Geometry: final body of the model. Coordinates: model frame, mm. A direction names the side the tool comes from. Round coordinates to 2 decimals unless told otherwise and drop trailing zeros. Loops run counter-clockwise (first coordinate to the right, second up) from the corner with the lowest first, then second, coordinate; pieces in that order, holes last. Notation, with made-up numbers: (74, 0) -> (102, 0) arc R16 ccw to (102, 12) -> close; hole circle Ø6 at (4, 66). An arc over 180 degrees is marked (long way). Answer in a Markdown table with one row per item.
Autodesk Inventor part; units mm, degrees
ref_plane "YZ Plane" through (0, 0, 0) normal (1, 0, 0) x (0, 1, 0)
ref_plane "XZ Plane" through (0, 0, 0) normal (0, 1, 0) x (-1, 0, 0)
ref_plane "XY Plane" through (0, 0, 0) normal (0, 0, 1) x (1, 0, 0)
sketch "Sketch_15" plane through (0, 0, 0) normal (1, 0, 0) x (0, 1, 0)
  line L0 (0, 30) -> (0, 0)
  line L1 (0, 0) -> (30, 0)
  line L2 (30, 0) -> (30, 4.0858)
  arc A0 (30, 4.0858) -> (29.7071, 4.7929) centre (29, 4.0858) ccw
  line L3 (29.7071, 4.7929) -> (4.7929, 29.7071)
  arc A1 (4.7929, 29.7071) -> (4.0858, 30) centre (4.0858, 29) ccw
  line L4 (4.0858, 30) -> (0, 30)
extrude "Extrusion1" add sketch "Sketch_15" along normal mid plane 20
sketch "Sketch_16" plane through (0, 0, 0) normal (1, 0, 0) x (0, 1, 0)
  line L0 (2.9278, 34.5) -> (4.5, 4.5)
  line L1 (4.5, 4.5) -> (34.5, 4.5)
  line L2 (34.5, 4.5) -> (34.5, 34.5)
  line L3 (34.5, 34.5) -> (2.9278, 34.5)
extrude "Extrusion2" cut sketch "Sketch_16" along normal mid plane 15
sketch "Sketch_17" plane through (0, 4.5, 0) normal (0, 1, 0) x (1, 0, 0)
  line L0 (-5.4209, -10.5) -> (-4.4687, -18.5299)
  arc A0 (-4.4687, -18.5299) -> (4.4687, -18.5299) centre (0, -18) ccw
  line L1 (4.4687, -18.5299) -> (5.4209, -10.5)
  line L2 (5.4209, -10.5) -> (-5.4209, -10.5)
extrude "Extrusion3" add sketch "Sketch_17" against normal blind 2.25
sketch "Sketch_2" plane through (0, 0, 0) normal (0, 0, 1) x (1, 0, 0)
  circle A0 centre (0, 18) radius 2.1
extrude "Extrusion4" cut sketch "Sketch_2" along normal blind 4.5
sketch "Sketch_9" plane through (0, 0, 0) normal (0, 0, 1) x (1, 0, 0)
  circle A0 centre (0, 10) radius 2.1
extrude "Extrusion5" cut sketch "Sketch_9" along normal blind 4.5
sketch "Sketch_3" plane through (0, 0, 0) normal (0, 1, 0) x (-1, 0, 0)
  circle A0 centre (0, 18) radius 2.1
extrude "Extrusion6" cut sketch "Sketch_3" along normal blind 4.5
sketch "Sketch_1" plane through (0, 0, 0) normal (0, 1, 0) x (-1, 0, 0)
  line L0 (10, 0) -> (10, 30)
  line L1 (10, 30) -> (-10, 30)
  line L2 (-10, 30) -> (-10, 0)
  line L3 (-10, 0) -> (10, 0)
extrude "Extrusion7" add sketch "Sketch_1" against normal blind 1
sketch "Sketch_4" plane through (0, 0, 0) normal (0, 1, 0) x (-1, 0, 0)
  line L0 (10, 0) -> (10, 30)
  line L1 (10, 30) -> (-10, 30)
  line L2 (-10, 30) -> (-10, 0)
  line L3 (-10, 0) -> (10, 0)
  arc A0 (3, 10.7) -> (2.7, 11) centre (2.7, 10.7) ccw
  line L4 (2.7, 11) -> (-2.7, 11)
  arc A1 (-2.7, 11) -> (-3, 10.7) centre (-2.7, 10.7) ccw
  line L5 (-3, 10.7) -> (-3, 5.3)
  arc A2 (-3, 5.3) -> (-2.7, 5) centre (-2.7, 5.3) ccw
  line L6 (-2.7, 5) -> (2.7, 5)
  arc A3 (2.7, 5) -> (3, 5.3) centre (2.7, 5.3) ccw
  line L7 (3, 5.3) -> (3, 10.7)
  arc A4 (3, 26.7) -> (2.7, 27) centre (2.7, 26.7) ccw
  line L8 (2.7, 27) -> (-2.7, 27)
  arc A5 (-2.7, 27) -> (-3, 26.7) centre (-2.7, 26.7) ccw
  line L9 (-3, 26.7) -> (-3, 24.3)
  arc A6 (-3, 24.3) -> (-2.7, 24) centre (-2.7, 24.3) ccw
  line L10 (-2.7, 24) -> (2.7, 24)
  arc A7 (2.7, 24) -> (3, 24.3) centre (2.7, 24.3) ccw
  line L11 (3, 24.3) -> (3, 26.7)
extrude "Extrusion8" cut sketch "Sketch_4" against normal blind 1
sketch "Sketch_10" plane through (0, 0, 0) normal (0, 0, 1) x (1, 0, 0)
  line L0 (-10, 0) -> (10, 0)
  line L1 (10, 0) -> (10, 30)
  line L2 (10, 30) -> (-10, 30)
  line L3 (-10, 30) -> (-10, 0)
extrude "Extrusion9" add sketch "Sketch_10" against normal blind 1
sketch "Sketch_11" plane through (0, 0, 0) normal (0, 0, 1) x (1, 0, 0)
  line L0 (-10, 0) -> (10, 0)
  line L1 (10, 0) -> (10, 30)
  line L2 (10, 30) -> (-10, 30)
  line L3 (-10, 30) -> (-10, 0)
  line L4 (0.5, 7) -> (2, 7)
  arc A0 (2, 7) -> (3, 8) centre (2, 8) ccw
  line L5 (3, 8) -> (3, 9.5)
  line L6 (3, 9.5) -> (2.0396, 9.5)
  arc A1 (0.5, 7.9604) -> (2.0396, 9.5) centre (0, 10) ccw
  line L7 (0.5, 7.9604) -> (0.5, 7)
  line L8 (0.5, 13) -> (0.5, 12.0396)
  arc A2 (2.0396, 10.5) -> (0.5, 12.0396) centre (0, 10) ccw
  line L9 (2.0396, 10.5) -> (3, 10.5)
  line L10 (3, 10.5) -> (3, 12)
  arc A3 (3, 12) -> (2, 13) centre (2, 12) ccw
  line L11 (2, 13) -> (0.5, 13)
  line L12 (-3, 9.5) -> (-3, 8)
  arc A4 (-3, 8) -> (-2, 7) centre (-2, 8) ccw
  line L13 (-2, 7) -> (-0.5, 7)
  line L14 (-0.5, 7) -> (-0.5, 7.9604)
  arc A5 (-2.0396, 9.5) -> (-0.5, 7.9604) centre (0, 10) ccw
  line L15 (-2.0396, 9.5) -> (-3, 9.5)
  line L16 (-3, 10.5) -> (-2.0396, 10.5)
  arc A6 (-0.5, 12.0396) -> (-2.0396, 10.5) centre (0, 10) ccw
  line L17 (-0.5, 12.0396) -> (-0.5, 13)
  line L18 (-0.5, 13) -> (-2, 13)
  arc A7 (-2, 13) -> (-3, 12) centre (-2, 12) ccw
  line L19 (-3, 12) -> (-3, 10.5)
extrude "Extrusion10" cut sketch "Sketch_11" against normal blind 1
properties part number "HBLFSN5-4hblfsn5"
Item 1: Section query C-C, the plane z = 2. Output: boundary loops of the cut face in (x, y).
Ans:
| item | result |
|---|---|
| outline | (-10, 0) -> (10, 0) -> (10, 30) -> (-10, 30) -> close; hole circle Ø4.2 at (0, 10); hole circle Ø4.2 at (0, 18) |
Item 2: Ray query, L1, parallel to Y at x = 0, z = 2.1; L2, parallel to X at y = 10.5, z = 1.5; L3, parallel to Z at x = 0, y = 1.4. Return the intervals inside material, ascending.
Ans:
| item | result |
|---|---|
| L1 | 0 to 7.9, 12.1 to 15.9, 20.1 to 30 |
| L2 | -10 to -2.04, 2.04 to 10 |
| L3 | 0 to 15.9, 20.1 to 30 |
Item 3: Section query A-A, the plane y = 18. Output: boundary loops of the cut face in (x, z), and give its area (3 significant figures).
Ans:
| item | result |
|---|---|
| outline | (-10, 0) -> (-2.1, 0) -> (-2.1, 4.5) -> (-7.5, 4.5) -> (-7.5, 16.5) -> (-10, 16.5) -> close; (2.1, 0) -> (10, 0) -> (10, 16.5) -> (7.5, 16.5) -> (7.5, 4.5) -> (2.1, 4.5) -> close |
| area | 131 mm2 |
Item 4: Mould query, pull axis X, two halves, no side actions, for faces 1 (the flat face through (3, 11.2, -0.5)), 2 (the flat face through (-2, 8, -1)), 3 (the flat face through (-0.5, 7.5, -0.5)). Classes: released by +X, released by -X, zero draft, split by the parting line, or undercut.
Ans:
| item | result |
|---|---|
| face 1 | released by +X |
| face 2 | zero draft |
| face 3 | undercut |
Item 5: Section query B-B, the plane x = 0. State how many separate pieces and enclosed holes the cut face has, and give its area (3 significant figures).
Ans:
| item | result |
|---|---|
| separate pieces | 4 |
| enclosed holes | 0 |
| area | 193 mm2 |
Item 6: Set-up query: faces 4 (the flat face through (-3, 8.8, -0.5)), 5 (the flat face through (-3, -0.5, 8)), 6 (the flat face through (0, 14, 4.5)), 7 (the flat face through (1.2, 7, -0.5)). Return all of +Z, -Z, +X, -X, +Y, -Y with unobstructed straight access to the full face (end or side cutting, diameter ignored); none if empty.
Ans:
| item | result |
|---|---|
| face 4 | -Z, -X, +Y, -Y |
| face 5 | +Z, -Z, -X, -Y |
| face 6 | +Z, +Y |
| face 7 | -Z, +X, -X, -Y |
Item 7: First-contact query: P1, Ø0.8, axis at x = 0.5, y = -0.5, coming from the -Z side; P2, Ø10, axis at x = 5, y = 20.5, coming from the -Z side; P3, Ø1, axis at x = 0.5, y = 11, coming from the -Z side; P4, Ø0.5, axis at x = -1, z = -0.5, coming from the -Y side. Flat tips, straight axial feed; report the tip coordinate or a pass-through.
Ans:
| item | result |
|---|---|
| P1 | z = 5 |
| P2 | z = 0 |
| P3 | through |
| P4 | y = 7 |
Item 8: Section query D-D, the plane y = 27.5. Output: boundary loops of the cut face in (x, z), and give its area (4 significant figures).
Ans:
| item | result |
|---|---|
| outline | (-10, 0) -> (10, 0) -> (10, 7) -> (7.5, 7) -> (7.5, 4.5) -> (-7.5, 4.5) -> (-7.5, 7) -> (-10, 7) -> close |
| area | 102.5 mm2 |
